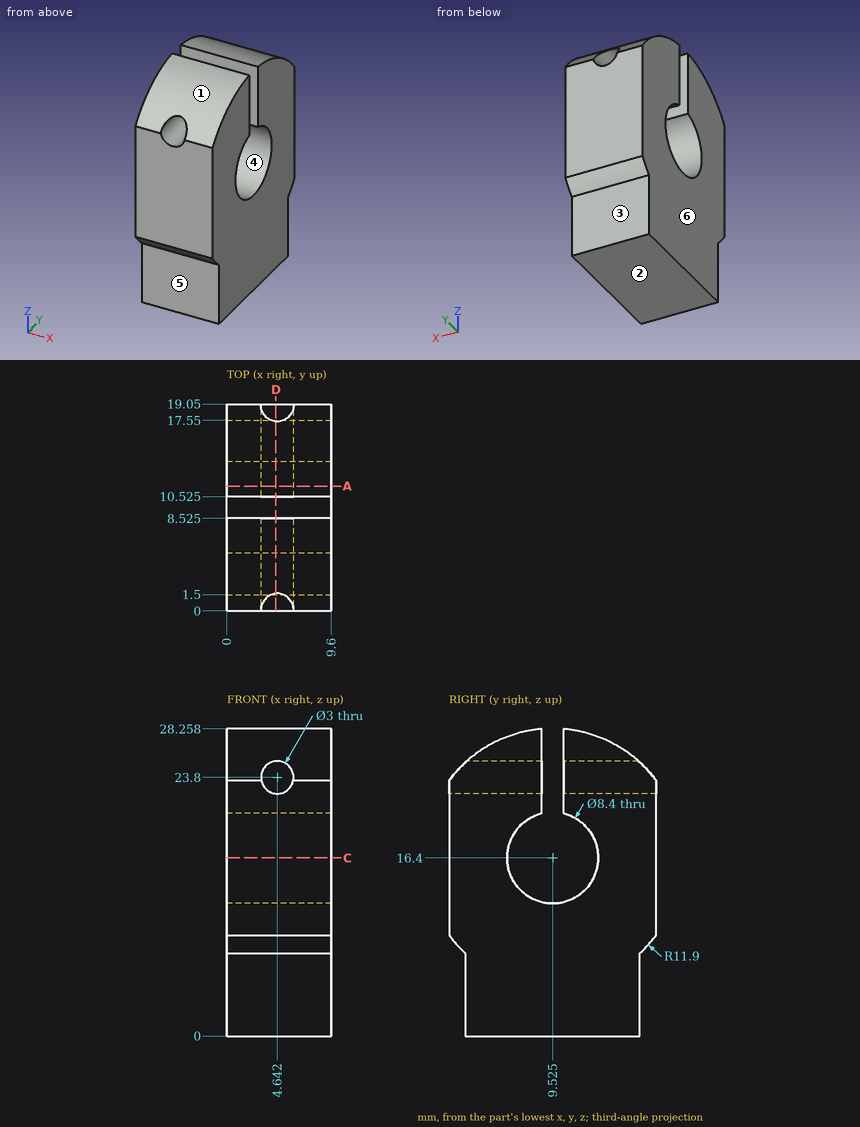
Verification items for this drawing (mm, ordinates from the low corner). A direction names the side the tool comes from. Coordinates: 2 decimals unless noted, no trailing zeros. Write each loop counter-clockwise with the first axis right and the second up, starting at its lowest first coordinate (ties: lowest second). Pieces come first, ordered by that corner, then holes. Notation, with made-up numbers: M 89,63.25 L 141,63.25 A26 cw 141,80.25 Z; hole C -38.75,36 d11. An arc over 180 degrees is marked long. Use one line per item in the form item = value. Start each with the question number.
1) Thickness scan on probe 1 along Y at (x, z) = (5, 16.4) (3 decimals); probe 2 along Z at (x, y) = (5.75, 7); probe 3 along X at (y, z) = (14.5, 23.8). Record the ranges inside material, lowest first. Write a range as from..to.
2) Release check for a two-part mould opening along Z. For the marked faces 1, 2, 3 and 4 record: pulls with the +Z half, pulls with the -Z half, needs draft (parallel to the pull), parting line crosses it, or undercut.
3) Section check D-D on x = 4.5. State how many separate pieces and enclosed holes the cut face has.
4) Set-up check for the marked faces 5 and 6: record each of +Z, -Z, +X, -X, +Y, -Y from which the full face is reachable in a straight line by a thin tool's end or side.
5) Section check C-C on z = 16.4. Enter the section's corners in (x, y) (3 decimals), and give its area (3 significant figures).
6) Section check A-A on y = 11.5. Enter the section's corners in (x, z) (1 decimal), and give its area (3 significant figures).
7) Go/stop test with flat-tipped pins: pin 1 Ø5 at (x, z) = (4.64, 23.8) entering from -Y; pin 2 Ø4 at (x, z) = (2.5, 3.5) entering from -Y; pin 3 Ø4 at (x, z) = (4, 5) entering from +Y; pin 4 Ø2.5 at (x, z) = (3, 25.5) entering from -Y. Record where each tip stops, or that it passes through.
Responses:
q1.probe_1 = 0..5.325, 13.725..19.05
q1.probe_2 = 0..13.04, 19.76..22.79, 24.81..28.03
q1.probe_3 = 0..3.14, 6.14..9.6
q2.face_1 = pulls with the +Z half
q2.face_2 = pulls with the -Z half
q2.face_3 = needs draft
q2.face_4 = undercut
q3.separate_pieces = 3
q3.enclosed_holes = 0
q4.face_5 = -Z, +X, -X, -Y
q4.face_6 = +Z, -Z, -X, +Y, -Y
q5.outline = M 0,0 L 9.6,0 L 9.6,5.325 L 0,5.325 Z; M 0,13.725 L 9.6,13.725 L 9.6,19.05 L 0,19.05 Z
q5.area = 102 mm2
q6.outline = M 0,0 L 9.6,0 L 9.6,12.7 L 0,12.7 Z; M 0,20.1 L 9.6,20.1 L 9.6,28.1 L 0,28.1 Z; hole C 4.6,23.8 d3
q6.area = 192 mm2
q7.pin_1 = 0
q7.pin_2 = 1.5
q7.pin_3 = 17.55
q7.pin_4 = 0.58
